Verification items for the finished model (mm, model axes). A direction names the side the tool comes from. Round coordinates to 2 decimals unless told otherwise and drop trailing zeros. Loops run counter-clockwise (first coordinate to the right, second up) from the corner with the lowest first, then second, coordinate; pieces in that order, holes last. Notation, with made-up numbers: (29, 14.5) -> (77, 14.5) arc R10 ccw to (77, 23.5) -> close; hole circle Ø2 at (56.25, 15). An arc over 180 degrees is marked (long way). Write item = value, one per line.
```python
from build123d import *

# Parameters (mm, degrees)
SKETCH_1_W          = 20
SKETCH_1_H          = 20
SKETCH_1_R          = 1.25
SKETCH_1_R_2        = 3
EXTRUDE_1_DEPTH     = 12
SKETCH_2_R          = 7.5
CUT_EXTRUDE_1_DEPTH = 5.2
CUT_EXTRUDE_2_DEPTH = 3


with BuildPart() as part:
    # 스케치1 → 보스-돌출1 (new body)
    with BuildSketch(Plane.XY):
        Rectangle(SKETCH_1_W, SKETCH_1_H)
        with Locations((-7.5, 7.5)):
            Circle(SKETCH_1_R, mode=Mode.SUBTRACT)
        with Locations((7.5, 7.5)):
            Circle(SKETCH_1_R, mode=Mode.SUBTRACT)
        with Locations((-7.5, -7.5)):
            Circle(SKETCH_1_R, mode=Mode.SUBTRACT)
        with Locations((7.5, -7.5)):
            Circle(SKETCH_1_R, mode=Mode.SUBTRACT)
        Circle(SKETCH_1_R_2, mode=Mode.SUBTRACT)
    extrude(amount=EXTRUDE_1_DEPTH)

    # 스케치2 → 컷-돌출1 (cut)
    with BuildSketch(Plane(origin=(0, 0, 0), x_dir=(-1, 0, 0), z_dir=(0, 0, -1))):
        Circle(SKETCH_2_R)
    extrude(amount=-CUT_EXTRUDE_1_DEPTH, mode=Mode.SUBTRACT)

    # 스케치3 → 컷-돌출2 (cut)
    with BuildSketch(Plane.XY.offset(12)):
        with BuildLine():
            Line((-10, -10), (-5, -10))
            Line((-5, -10), (-5, -7.5))
            ThreePointArc((-5, -7.5), (-5.732233047, -5.732233047), (-7.5, -5))
            Line((-7.5, -5), (-10, -5))
            Line((-10, -5), (-10, -10))
        make_face()
        with BuildLine():
            Line((-7.5, 5), (-10, 5))
            Line((-10, 5), (-10, 10))
            Line((-10, 10), (-5, 10))
            Line((-5, 10), (-5, 7.5))
            ThreePointArc((-5, 7.5), (-5.732233047, 5.732233047), (-7.5, 5))
        make_face()
        with BuildLine():
            Line((7.5, 5), (10, 5))
            Line((10, 5), (10, 10))
            Line((10, 10), (5, 10))
            Line((5, 10), (5, 7.5))
            ThreePointArc((5, 7.5), (5.732233047, 5.732233047), (7.5, 5))
        make_face()
        with BuildLine():
            Line((7.5, -5), (10, -5))
            Line((10, -5), (10, -10))
            Line((10, -10), (5, -10))
            Line((5, -10), (5, -7.5))
            ThreePointArc((5, -7.5), (5.732233047, -5.732233047), (7.5, -5))
        make_face()
    extrude(amount=-CUT_EXTRUDE_2_DEPTH, mode=Mode.SUBTRACT)


solid = part.part
```
(1) Set-up check for faces 1 (the face through (-5, -9, 11)), 2 (the face through (-3.2, 0.1, 5.2)), 3 (the face through (9, -5, 11)), 4 (the face through (-9, 5, 11)), 5 (the face through (5, 9, 11)): record each of +Z, -Z, +X, -X, +Y, -Y from which the full face is reachable in a straight line by a thin tool's end or side.
Filled sheet:
face_1 = +Z, -X, -Y
face_2 = -Z
face_3 = +Z, +X, -Y
face_4 = +Z, -X, +Y
face_5 = +Z, +X, +Y
(2) Sectioned sample at B-B, the plane z = 9.25. Record the cut outline in (x, y), and give its area (3 significant figures).
Filled sheet:
outline = (-10, -5) -> (-7.5, -5) arc R2.5 cw to (-5, -7.5) -> (-5, -10) -> (5, -10) -> (5, -7.5) arc R2.5 cw to (7.5, -5) -> (10, -5) -> (10, 5) -> (7.5, 5) arc R2.5 cw to (5, 7.5) -> (5, 10) -> (-5, 10) -> (-5, 7.5) arc R2.5 cw to (-7.5, 5) -> (-10, 5) -> close; hole circle Ø6 at (0, 0)
area = 277 mm2
(3) Sectioned sample at D-D, the plane x = 8. Record the cut outline in (y, z), and give its area (3 significant figures).
Filled sheet:
outline = (-10, 0) -> (-8.65, 0) -> (-8.65, 9) -> (-10, 9) -> close; (-6.35, 0) -> (6.35, 0) -> (6.35, 9) -> (5, 9) -> (5, 12) -> (-5, 12) -> (-5, 9) -> (-6.35, 9) -> close; (8.65, 0) -> (10, 0) -> (10, 9) -> (8.65, 9) -> close
area = 169 mm2
(4) Material ranges on probe 1 along X at (y, z) = (7.5, 5.75); probe 2 along Y at (x, z) = (0, 2.45), recorded low to high. Write a range as from..to.
Filled sheet:
probe_1 = -10..-8.75, -6.25..6.25, 8.75..10
probe_2 = -10..-7.5, 7.5..10
(5) Go/stop test with flat-tipped pins: pin 1 Ø3 at (x, y) = (-7.5, 7.5) entering from +Z; pin 2 Ø0.8 at (y, z) = (9.5, 11) entering from -X; pin 3 Ø1.2 at (y, z) = (-8.5, 11) entering from +X. Record where each tip stops, or that it passes through.
Filled sheet:
pin_1 = 9
pin_2 = -5
pin_3 = 5
(6) Draft check along X on faces 6 (the face through (6.25, -7.45, 4.44)), 7 (the face through (-10, 0, 6)), 8 (the face through (8, 9, 9)). Enter one of: released by +X, released by -X, zero draft, split by the parting line, or undercut.
Filled sheet:
face_6 = undercut
face_7 = released by -X
face_8 = zero draft
(7) Sectioned sample at A-A, the plane x = 0. Record the cut outline in (y, z).
Filled sheet:
outline = (-10, 0) -> (-7.5, 0) -> (-7.5, 5.2) -> (-3, 5.2) -> (-3, 12) -> (-10, 12) -> close; (3, 5.2) -> (7.5, 5.2) -> (7.5, 0) -> (10, 0) -> (10, 12) -> (3, 12) -> close
